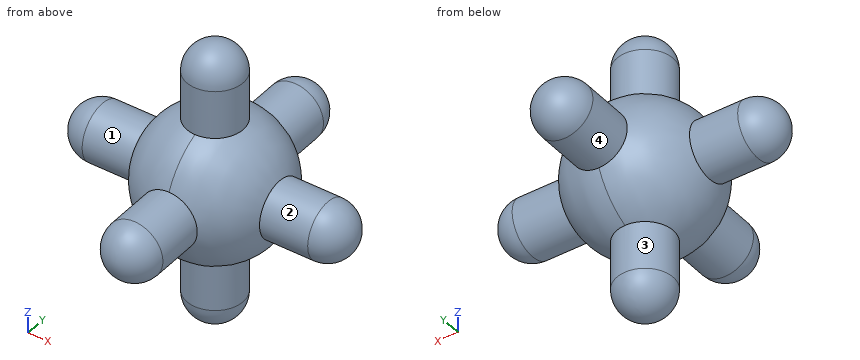
from build123d import *

# Parameters (mm, degrees)
SKETCH1_R           = 25
BOSS_EXTRUDE1_DEPTH = 25
FILLET1_R           = 25
SKETCH2_R           = 10
BOSS_EXTRUDE2_DEPTH = 50
FILLET2_R           = 10
SKETCH3_R           = 10
BOSS_EXTRUDE3_DEPTH = 50
FILLET3_R           = 10
SKETCH4_R           = 10
BOSS_EXTRUDE4_DEPTH = 50
FILLET4_R           = 10


with BuildPart() as part:
    # Sketch1 → Boss-Extrude1 (new, symmetric)
    with BuildSketch(Plane(origin=(0, 0, 0), x_dir=(0, 0, -1), z_dir=(1, 0, 0))):
        Circle(SKETCH1_R)
    extrude(amount=BOSS_EXTRUDE1_DEPTH, both=True)

    # Fillet1
    fillet1_edges = [part.edges().sort_by_distance(p)[0] for p in [
        (-25, 0, 25),
        (25, 0, 25),
    ]]
    fillet(fillet1_edges, radius=FILLET1_R - 0.0001)  # a hair under: the kernel refuses the full size

    # Sketch2 → Boss-Extrude2 (add, symmetric)
    with BuildSketch(Plane(origin=(0, 0, 0), x_dir=(0, 0, -1), z_dir=(1, 0, 0))):
        with Locations(Location((0, 0, 0), (0, 0, 180))):
            Circle(SKETCH2_R)
    extrude(amount=BOSS_EXTRUDE2_DEPTH, both=True)

    # Fillet2
    fillet2_edges = [part.edges().sort_by_distance(p)[0] for p in [
        (50, 0, -10),
        (-50, 0, -10),
    ]]
    fillet(fillet2_edges, radius=FILLET2_R)

    # Sketch3 → Boss-Extrude3 (add, symmetric)
    with BuildSketch(Plane.XY):
        with Locations(Location((0, 0, 0), (0, 0, 90))):
            Circle(SKETCH3_R)
    extrude(amount=BOSS_EXTRUDE3_DEPTH, both=True)

    # Fillet3
    fillet3_edges = [part.edges().sort_by_distance(p)[0] for p in [
        (0, -10, -50),
        (0, -10, 50),
    ]]
    fillet(fillet3_edges, radius=FILLET3_R)

    # Sketch4 → Boss-Extrude4 (add, symmetric)
    with BuildSketch(Plane(origin=(0, 0, 0), x_dir=(1, 0, 0), z_dir=(0, 1, 0))):
        with Locations(Location((0, 0, 0), (0, 0, 270))):
            Circle(SKETCH4_R)
    extrude(amount=BOSS_EXTRUDE4_DEPTH, both=True)

    # Fillet4
    fillet4_edges = [part.edges().sort_by_distance(p)[0] for p in [
        (0, -50, -10),
        (0, 50, -10),
    ]]
    fillet(fillet4_edges, radius=FILLET4_R)


solid = part.part
The listing builds one solid part. Answer for the finished solid, in the listing's coordinates (mm). Face numbers are marked on the shaded views. A direction names the side the tool comes from. Round coordinates to 2 decimals unless told otherwise and drop trailing zeros. Write each loop counter-clockwise with the first axis right and the second up, starting at its lowest first coordinate (ties: lowest second). Pieces come first, ordered by that corner, then holes. Notation, with made-up numbers: M 78.25,20 L 101.25,20 A36 ccw 101.25,58 Z; hole C 53,57 d6. An arc over 180 degrees is marked long. Write each question's results on one line, items separated by ' | '. Start each with the question number.
Item 1: For the marked faces 1, 2, 3 and 4, determine the directions among +Z, -Z, +X, -X, +Y, -Y from which every point of the face is accessible in a straight line to the end or side of a thin tool.
Item 2: Straight lines are drawn through the part: L1, parallel to X at y = -40, z = 0.5; L2, parallel to X at y = 27, z = -7; L3, parallel to Z at x = -27, y = -5.5. For each, find the intervals that lie inside material, in ascending order. Write a range as [from, to].
Item 3: Flat-ended cylindrical pins translate along their axes: pin 1 Ø8 at (y, z) = (9, 26.5) entering from +X; pin 2 Ø10 at (x, z) = (31.5, 2) entering from +Y; pin 3 Ø3 at (y, z) = (-8.5, 34.5) entering from +X. Find the tip coordinate at first contact, or state that the pin passes through.
Item 4: A cutting plane is placed at A-A on z = -25. Write down the section's boundary in (x, y).
Check sheet entries:
1) face 1: -X | face 2: +X | face 3: -Z | face 4: +Y
2) L1: [-9.99, 9.99] | L2: [-7.14, 7.14] | L3: [-8.35, 8.35]
3) pin 1: x = 8.66 | pin 2: y = 10 | pin 3: x = 7.14
4) outline: C 0,0 d20
